```python
from build123d import *

# Parameters (mm, degrees)
SKETCH1_W           = 20
SKETCH1_H           = 16
SKETCH1_R           = 3
SKETCH1_R_2         = 1.5
BOSS_EXTRUDE1_DEPTH = 11.5
CUT_EXTRUDE1_DEPTH  = 17
SKETCH3_R           = 1.25
SKETCH3_R_2         = 1
CUT_EXTRUDE2_DEPTH  = 3
CHAMFER1_SIZE       = 0.5


with BuildPart() as part:
    # Sketch1 → Boss-Extrude1 (new body)
    with BuildSketch(Plane(origin=(0, 0, 0), x_dir=(1, 0, 0), z_dir=(0, 1, 0))):
        Rectangle(SKETCH1_W, SKETCH1_H)
        with Locations((5.5, 0)):
            Circle(SKETCH1_R, mode=Mode.SUBTRACT)
        with Locations((-7.5, 0)):
            Circle(SKETCH1_R_2, mode=Mode.SUBTRACT)
    extrude(amount=BOSS_EXTRUDE1_DEPTH)

    # Sketch2 → Cut-Extrude1 (cut, through all)
    with BuildSketch(Plane.XY.offset(8)):
        with BuildLine():
            Line((-10, 5), (-4.328427125, 5))
            ThreePointArc((-4.328427125, 5), (1.5, 4), (-4.328427125, 3))
            Line((-4.328427125, 3), (-10, 3))
            Line((-10, 3), (-10, 5))
        make_face()
    extrude(amount=-CUT_EXTRUDE1_DEPTH, mode=Mode.SUBTRACT)

    # Sketch3 → Cut-Extrude2 (cut)
    with BuildSketch(Plane.XY.offset(8)):
        with Locations((6.5, 4.8)):
            Circle(SKETCH3_R)
        with Locations((8, 2)):
            Circle(SKETCH3_R_2)
    extrude(amount=-CUT_EXTRUDE2_DEPTH, mode=Mode.SUBTRACT)

    # Chamfer1
    chamfer1_edges = [part.edges().sort_by_distance(p)[0] for p in [
        (10, 11.5, 0),
        (0, 11.5, -8),
        (-10, 1.5, -8),
        (-10, 1.5, 8),
        (-10, 11.5, 0),
        (0, 0, -8),
        (10, 0, 0),
        (0, 0, 8),
        (-10, 0, 0),
        (0, 11.5, 8),
        (-10, 8.25, -8),
        (10, 5.75, -8),
        (10, 5.75, 8),
        (-10, 8.25, 8),
    ]]
    chamfer(chamfer1_edges, length=CHAMFER1_SIZE)


solid = part.part
```
Design review of the part built by this model. Coordinates are the model's own, in mm. A direction names the side the tool comes from. Give positions to 0.01 mm unless a question says otherwise; leave off trailing zeros. Write each loop counter-clockwise with the first axis right and the second up, starting at its lowest first coordinate (ties: lowest second). Pieces come first, ordered by that corner, then holes.
(1) Add section D-D (x = 6.5). Give the boundary of the cut face in (y, z), and give its area (3 significant figures).
Checked values:
outline: (0, -7.5) - (0.5, -8) - (11, -8) - (11.5, -7.5) - (11.5, -2.83) - (0, -2.83) - close; (0, 2.83) - (11.5, 2.83) - (11.5, 7.5) - (11, 8) - (6.05, 8) - (6.05, 5) - (3.55, 5) - (3.55, 8) - (0.5, 8) - (0, 7.5) - close
area: 111 mm2
(2) Add section B-B (x = -7.5). Give the boundary of the cut face in (y, z), and give its area (3 significant figures).
Checked values:
outline: (0, -7.5) - (0.5, -8) - (3, -8) - (3, -1.5) - (0, -1.5) - close; (0, 1.5) - (3, 1.5) - (3, 8) - (0.5, 8) - (0, 7.5) - close; (5, -8) - (11, -8) - (11.5, -7.5) - (11.5, -1.5) - (5, -1.5) - close; (5, 1.5) - (11.5, 1.5) - (11.5, 7.5) - (11, 8) - (5, 8) - close
area: 123 mm2
(3) Add section A-A (y = 5.5). Give the boundary of the cut face in (x, z), and give its area (3 significant figures).
Checked values:
outline: (-10, -7.5) - (-9.5, -8) - (-4.1, -8) - (-4.1, 8) - (-9.5, 8) - (-10, 7.5) - close; (1.1, -8) - (9.5, -8) - (10, -7.5) - (10, 7.5) - (9.5, 8) - (7.54, 8) - (7.54, 5) - (5.46, 5) - (5.46, 8) - (1.1, 8) - close; hole circle Ø3 at (-7.5, 0); hole circle Ø6 at (5.5, 0)
area: 195 mm2
(4) Wall thickness on line 1 along Z through (x, y) = (-7.5, 8); line 2 along X through (y, z) = (6.5, 0); line 3 along X through (y, z) = (2.2, 0): over which ranges is each line inside the solid? List them lowest first.
Checked values:
line 1: z = -8 to -1.5, 1.5 to 8
line 2: x = -10 to -9, -6 to -3.16, 0.16 to 2.5, 8.5 to 10
line 3: x = -10 to -9, -6 to -3.9, 0.9 to 2.5, 8.5 to 10
(5) Clearance check with a flat-ended pin moving along its axis: pin 1 Ø2.5 at (x, z) = (-7.5, 0) entering from +Y. State where the tip first meets the part, or that it passes through.
Checked values:
pin 1: passes through
(6) Mouldability with a two-part tool opening along Y and no side actions: class faces 1 (the face through (0, 7, 8)), 2 (the face through (5.25, 4.85, 6.52)), 3 (the face through (0, 11.5, 0)) as +Y half, -Y half, draft (parallel to the pull), parting line (faces both ways), or undercut.
Checked values:
face 1: draft
face 2: undercut
face 3: +Y half
(7) Add section C-C (y = 10.25). Give the boundary of the cut face in (x, z), and give its area (3 significant figures).
Checked values:
outline: (-10, -7.5) - (-9.5, -8) - (9.5, -8) - (10, -7.5) - (10, 7.5) - (9.5, 8) - (-9.5, 8) - (-10, 7.5) - close; hole circle Ø3 at (-7.5, 0); hole circle Ø6 at (5.5, 0)
area: 284 mm2
(8) Tool access review of faces 4 (the face through (8, 2, 5)), 5 (the face through (0, 7, -8)), 6 (the face through (-7, 5, 2)): name each direction out of +Z, -Z, +X, -X, +Y, -Y from which nothing blocks a thin tool from reaching the whole face with its end or side.
Checked values:
face 4: +Z
face 5: -Z, +X, -X, +Y, -Y
face 6: +Z, -Z, -X
